from build123d import *

# Parameters (mm, degrees)
BOSS_EXTRUDE1_DEPTH = 60
CIRPATTERN1_COUNT   = 4


with BuildPart() as part:
    # Sketch3 → Boss-Extrude1 (new, symmetric)
    with BuildSketch(Plane.XY):
        with BuildLine():
            Line((-4.503841895, 3.156803476), (-3.14772708, 1.530298739))
            ThreePointArc((-3.14772708, 1.530298739), (-3.410794979, 0.785160882), (-3.5, 0))
            Line((-3.5, 0), (-5.5, 0))
            Line((-5.5, 0), (-6, 0.866025404))
            Line((-6, 0.866025404), (-6, 3.996841995))
            ThreePointArc((-6, 3.996841995), (-6.038060234, 4.188183711), (-6.146446609, 4.350395385))
            Line((-6.146446609, 4.350395385), (-9.917104615, 8.121053391))
            ThreePointArc((-9.917104615, 8.121053391), (-10.079316289, 8.229439766), (-10.270658005, 8.2675))
            Line((-10.270658005, 8.2675), (-12.29, 8.2675))
            ThreePointArc((-12.29, 8.2675), (-12.643553391, 8.121053391), (-12.79, 7.7675))
            Line((-12.79, 7.7675), (-12.79, 4.5))
            ThreePointArc((-12.79, 4.5), (-12.936446609, 4.146446609), (-13.29, 4))
            Line((-13.29, 4), (-14.5, 4))
            Line((-14.5, 4), (-14.5, 4.5))
            Line((-14.5, 4.5), (-15, 4.5))
            Line((-15, 4.5), (-15, 12.968))
            ThreePointArc((-15, 12.968), (-14.404840979, 14.404840979), (-12.968, 15))
            Line((-12.968, 15), (-4.5, 15))
            Line((-4.5, 15), (-4.5, 14.5))
            Line((-4.5, 14.5), (-4, 14.5))
            Line((-4, 14.5), (-4, 13.29))
            ThreePointArc((-4, 13.29), (-4.146446609, 12.936446609), (-4.5, 12.79))
            Line((-4.5, 12.79), (-7.7675, 12.79))
            ThreePointArc((-7.7675, 12.79), (-8.121053391, 12.643553391), (-8.2675, 12.29))
            Line((-8.2675, 12.29), (-8.2675, 10.270658005))
            ThreePointArc((-8.2675, 10.270658005), (-8.229439766, 10.079316289), (-8.121053391, 9.917104615))
            Line((-8.121053391, 9.917104615), (-4.350395385, 6.146446609))
            ThreePointArc((-4.350395385, 6.146446609), (-4.188183711, 6.038060234), (-3.996841995, 6))
            Line((-3.996841995, 6), (-0.866025404, 6))
            Line((-0.866025404, 6), (0, 5.5))
            Line((0, 5.5), (0, 3.5))
            ThreePointArc((0, 3.5), (-0.785160882, 3.410794979), (-1.530298739, 3.14772708))
            Line((-1.530298739, 3.14772708), (-3.156803476, 4.503841895))
            ThreePointArc((-3.156803476, 4.503841895), (-3.889087297, 3.889087297), (-4.503841895, 3.156803476))
        make_face()
        with BuildLine():
            Line((-12.705, 9.5135), (-10.5135, 9.5135))
            ThreePointArc((-10.5135, 9.5135), (-9.806393219, 9.806393219), (-9.5135, 10.5135))
            Line((-9.5135, 10.5135), (-9.5135, 12.705))
            ThreePointArc((-9.5135, 12.705), (-9.806393219, 13.412106781), (-10.5135, 13.705))
            Line((-10.5135, 13.705), (-12.705, 13.705))
            ThreePointArc((-12.705, 13.705), (-13.412106781, 13.412106781), (-13.705, 12.705))
            Line((-13.705, 12.705), (-13.705, 10.5135))
            ThreePointArc((-13.705, 10.5135), (-13.412106781, 9.806393219), (-12.705, 9.5135))
        make_face(mode=Mode.SUBTRACT)
    boss_extrude1 = extrude(amount=BOSS_EXTRUDE1_DEPTH, both=True)

    # CirPattern1: Boss-Extrude1 ×4 about axis
    cirpattern1_axis = Axis((0, 0, 0), (0, 0, 1))
    for i in range(1, CIRPATTERN1_COUNT):
        add(boss_extrude1.rotate(cirpattern1_axis, i * 360 / CIRPATTERN1_COUNT))


solid = part.part
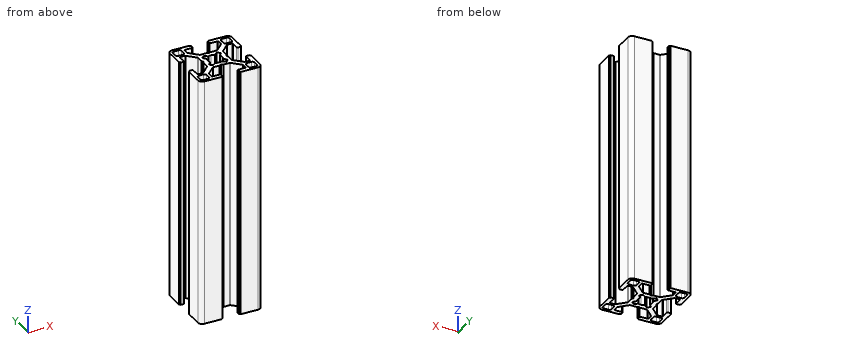
Geometry check sheet. Reference: the model listing, model coordinates, mm. Give positions to 0.01 mm unless a question says otherwise; leave off trailing zeros. Use a Markdown table: item, result.
Item 1: Material ranges on line 1 along X through (y, z) = (-10.5, -43); line 2 along Y through (x, z) = (-12.5, 44.5) (1 decimal), recorded low to high.
Answers follow:
| item | result |
|---|---|
| line 1 | x = -15 to -13.7, -9.51 to -8.27, 8.27 to 9.51, 13.7 to 15 |
| line 2 | y = -15 to -13.7, -9.5 to -8.2, 8.2 to 9.5, 13.7 to 15 |
Item 2: Depth check by flat-ended pin: P1, Ø0.6, axis at x = -4, z = 7, coming from the -Y side; P2, Ø2.5, axis at y = 1.5, z = 27, coming from the -X side. Enter the tip coordinate at first touch or a pass-through.
Answers follow:
| item | result |
|---|---|
| P1 | stops at y = -14.5 |
| P2 | stops at x = -6 |
Item 3: Section check A-A (z = 13). State how many separate pieces and enclosed holes the cut face has, and give its area (3 significant figures).
Answers follow:
| item | result |
|---|---|
| separate pieces | 1 |
| enclosed holes | 5 |
| area | 317 mm2 |
